Build history of the part. All positions in model axes, mm. A direction names the side the tool comes from. Give positions to 0.01 mm unless a question says otherwise; leave off trailing zeros. Order: outer loops, then holes, each group sorted by start corner. A loop starts at its lowest first (then second) coordinate and runs counter-clockwise, first axis right, second up. Notation, with made-up numbers: (35.5, 73.25) - (80.5, 73.25) arc R22 cw to (80.5, 81.25) - close; hole circle Ø3 at (77, -14.5). An arc over 180 degrees is marked (long way). One line per item, written item: value.
```python
from build123d import *

# Parameters (mm, degrees)
F1_DEPTH = 63.5
F2_DEPTH = 25.4
F3_DEPTH = 7.9375
F5_R     = 6.35


with BuildPart() as f1:
    # F0 (on Front) → F1 (new body, symmetric)
    with BuildSketch(Plane.XZ):
        Polygon((22.225, 9.525), (-41.275, 9.525), (-41.275, -9.525), (41.275, -9.525), (41.275, 9.525), align=None)
    extrude(amount=F1_DEPTH, both=True)

    # F0 (on Front) → F2 (join, symmetric)
    with BuildSketch(Plane.XZ):
        with BuildLine():
            Line((22.225, 26.3652), (22.225, 9.525))
            Line((22.225, 9.525), (41.275, 9.525))
            Line((41.275, 9.525), (41.275, 26.3652))
            ThreePointArc((41.275, 26.3652), (46.110667, 38.039533), (57.785, 42.8752))
            Line((57.785, 42.8752), (60.325, 42.8752))
            Line((60.325, 42.8752), (60.325, 61.9252))
            Line((60.325, 61.9252), (57.785, 61.9252))
            add(Edge.make_bspline(
                [(54.999193, 61.815911), (55.93158, 61.863075), (56.860354, 61.899531), (57.785, 61.9252)],
                knots=[109.33874, 109.33874, 109.33874, 109.33874, 112.065448, 112.065448, 112.065448, 112.065448], degree=3))
            ThreePointArc((54.999193, 61.815911), (31.673921, 50.504901), (22.225, 26.3652))
        make_face()
        Polygon((60.325, 66.675), (60.325, 61.9252), (60.325, 42.8752), (60.325, 38.1), (111.125, 38.1), (111.125, 66.675), align=None)
    extrude(amount=F2_DEPTH, both=True)

    # F0 (on Front) → F3 (join, symmetric)
    with BuildSketch(Plane.XZ):
        with BuildLine():
            add(Edge.make_bspline(
                [(-41.275, 9.525), (-25.584794, 40.814355), (17.611256, 59.924649), (54.999193, 61.815911)],
                knots=[0, 0, 0, 0, 109.33874, 109.33874, 109.33874, 109.33874], degree=3))
            Line((-41.275, 9.525), (22.225, 9.525))
            Line((22.225, 9.525), (22.225, 26.3652))
            ThreePointArc((22.225, 26.3652), (31.673921, 50.504901), (54.999193, 61.815911))
        make_face()
    extrude(amount=F3_DEPTH, both=True)

    # F0 (on Front) → F4 (revolve)
    with BuildSketch(Plane.XZ):
        Polygon((60.325, 66.675), (60.325, 61.9252), (60.325, 42.8752), (60.325, 38.1), (111.125, 38.1), (111.125, 66.675), align=None)
    revolve(axis=Axis((111.125, 0, 52.3875), (0, 0, -1)))

    # F5
    f5_edges = [f1.edges().sort_by_distance(p)[0] for p in [
        (41.275, 63.5, 0),
        (-41.275, 63.5, 0),
        (41.275, -63.5, 0),
        (-41.275, -63.5, 0),
    ]]
    fillet(f5_edges, radius=F5_R)


solid = f1.part
```
(1) Slice it at D-D, the plane y = 44. Give the cut face in (x, z) (3 decimals), and give its area (3 significant figures).
Completed:
outline: (-41.275, -9.525) - (41.275, -9.525) - (41.275, 9.525) - (-41.275, 9.525) - close; (85.735, 38.1) - (136.515, 38.1) - (136.515, 66.675) - (85.735, 66.675) - close
area: 3,020 mm²
(2) 3-axis set-ups, long thin cutter, end or side, ignore diameter. For faces 1 (the face through (31.93, 16.55, 50.78)), 2 (the face through (112, 1, 38.1)), 3 (the face through (60.325, 0, 41)), 4 (the face through (60.325, 0, 64)): which of +Z, -Z, +X, -X, +Y, -Y reach the whole face in a straight line?
Completed:
face 1: +Z, -X, +Y
face 2: -Z, +X, +Y, -Y
face 3: -Z, +Y, -Y
face 4: +Z, -X, +Y, -Y
(3) Slice it at B-B, the plane y = -34. Give the cut face in (x, z) (3 decimals), and give its area (3 significant figures).
Completed:
outline: (-41.275, -9.525) - (41.275, -9.525) - (41.275, 9.525) - (-41.275, 9.525) - close; (73.381, 38.1) - (148.869, 38.1) - (148.869, 66.675) - (73.381, 66.675) - close
area: 3,730 mm²
(4) Drill centre lines: line 1 (Y direction, x = -24, z = 26); line 2 (Z direction, x = 90, y = -13) (3 decimals); line 3 (X direction, y = -17, z = 8.5) (3 decimals). Where is each one in solid material? Low to high.
Completed:
line 1: -7.94 to 7.94
line 2: 38.1 to 66.675
line 3: -41.275 to 41.275
(5) Slice it at C-C, the plane y = -54.5. Give the cut face in (x, z) (3 decimals).
Completed:
outline: (-41.275, -9.525) - (41.275, -9.525) - (41.275, 9.525) - (-41.275, 9.525) - close
(6) Pull direction X, two halves, no side cores. Call faces 5 (the face through (-39.365, -61.689, -0.133)), 6 (the face through (45.98, -0.36, 37.91)), 7 (the face through (1, 35, 9.525)): +X half, -X half, draft (parallel to the pull), parting line (faces both ways), or undercut.
Completed:
face 5: -X half
face 6: undercut
face 7: draft
(7) Slice it at A-A, the plane z = 6.5. Give the cut face in (x, y) (3 decimals), and give its area (3 significant figures).
Completed:
outline: (-41.275, -57.15) arc R6.35 ccw to (-34.925, -63.5) - (34.925, -63.5) arc R6.35 ccw to (41.275, -57.15) - (41.275, 57.15) arc R6.35 ccw to (34.925, 63.5) - (-34.925, 63.5) arc R6.35 ccw to (-41.275, 57.15) - close
area: 10,400 mm²
(8) Pin check, flat tips, straight feed: P1, Ø2.5, axis at y = 6.5, z = 39.5, coming from the -X side; P2, Ø12, axis at x = 77, z = 48.5, coming from the -Y side; P3, Ø15.5, axis at x = 4, z = 37, coming from the -Y side. Stop position of each tip, or through.
Completed:
P1: x = -15.33
P2: y = -42.3
P3: y = -7.94
